Can you work these out from the model? Positions are in its coordinate system, mm. Face numbers are marked on the shaded views. A direction names the side the tool comes from. Round coordinates to 2 decimals unless told otherwise and drop trailing zeros. Loops run counter-clockwise (first coordinate to the right, second up) from the corner with the lowest first, then second, coordinate; pieces in that order, holes last. Notation, with made-up numbers: M 66.25,60.5 L 91.25,60.5 A5 cw 91.25,69.5 Z; hole C -18,57 d6. An arc over 180 degrees is marked long. Answer as CSV lines item,"result".
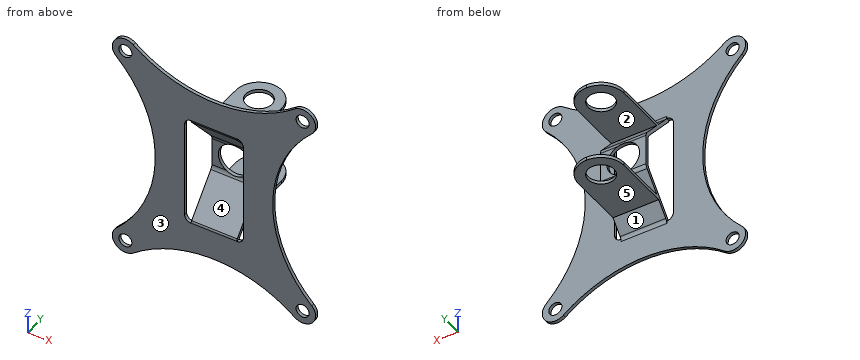
from build123d import *

# Parameters (mm, degrees)
BOSS_EXTRUDE1_DEPTH = 3.175
BOSS_EXTRUDE3_DEPTH = 22.225
SKETCH5_R           = 15.875
CUT_EXTRUDE1_DEPTH  = 35.925
SKETCH6_R           = 12.7
CUT_EXTRUDE2_DEPTH  = 79.375
FILLET1_R           = 6.35
SKETCH1_5_R         = 6.35
HOLES_DEPTH         = 92.0082


with BuildPart() as part:
    # Sketch1 → Boss-Extrude1 (new body)
    with BuildSketch(Plane(origin=(0, 0, 0), x_dir=(1, 0, 0), z_dir=(0, 1, 0))):
        with BuildLine():
            ThreePointArc((-78.393636364, 109.635915457), (-95.772926059, 108.027505481), (-95.134259734, 90.585636364))
            ThreePointArc((-95.134259734, 90.585636364), (-57.14685707, 0), (-95.134259734, -90.585636364))
            ThreePointArc((-95.134259734, -90.585636364), (-95.772926059, -108.027505481), (-78.393636364, -109.635915457))
            ThreePointArc((-78.393636364, -109.635915457), (0, -82.553070029), (78.393636364, -109.635915457))
            ThreePointArc((78.393636364, -109.635915457), (95.772926059, -108.027505481), (95.134259734, -90.585636364))
            ThreePointArc((95.134259734, -90.585636364), (57.14685707, 0), (95.134259734, 90.585636364))
            ThreePointArc((95.134259734, 90.585636364), (95.772926059, 108.027505481), (78.393636364, 109.635915457))
            ThreePointArc((78.393636364, 109.635915457), (0, 82.553070029), (-78.393636364, 109.635915457))
        make_face()
        with BuildLine():
            Line((-22.225, -53.975), (22.225, -53.975))
            ThreePointArc((22.225, -53.975), (26.715128061, -52.115128061), (28.575, -47.625))
            Line((28.575, -47.625), (28.575, 47.625))
            ThreePointArc((28.575, 47.625), (26.715128061, 52.115128061), (22.225, 53.975))
            Line((22.225, 53.975), (-22.225, 53.975))
            ThreePointArc((-22.225, 53.975), (-26.715128061, 52.115128061), (-28.575, 47.625))
            Line((-28.575, 47.625), (-28.575, -47.625))
            ThreePointArc((-28.575, -47.625), (-26.715128061, -52.115128061), (-22.225, -53.975))
        make_face(mode=Mode.SUBTRACT)
    extrude(amount=BOSS_EXTRUDE1_DEPTH)

    # Sketch4 → Boss-Extrude3 (add, symmetric)
    with BuildSketch(Plane(origin=(0, 0, 0), x_dir=(0, 0, -1), z_dir=(1, 0, 0))):
        with BuildLine():
            ThreePointArc((53.975, 0), (52.866902818, 0.199643612), (51.898159667, 0.773467316))
            Line((51.898159667, 0.773467316), (17.867550541, 30.203065368))
            ThreePointArc((17.867550541, 30.203065368), (15.930064238, 31.350712776), (13.713869875, 31.75))
            Line((13.713869875, 31.75), (-13.713869875, 31.75))
            ThreePointArc((-13.713869875, 31.75), (-15.930064238, 31.350712776), (-17.867550541, 30.203065368))
            Line((-17.867550541, 30.203065368), (-51.898159667, 0.773467316))
            ThreePointArc((-51.898159667, 0.773467316), (-52.866902818, 0.199643612), (-53.975, 0))
            Line((-53.975, 0), (-53.975, 3.175))
            Line((-53.975, 3.175), (-19.05, 33.378065368))
            ThreePointArc((-19.05, 33.378065368), (-17.112513698, 34.525712776), (-14.896319334, 34.925))
            Line((-14.896319334, 34.925), (14.896319334, 34.925))
            ThreePointArc((14.896319334, 34.925), (17.112513698, 34.525712776), (19.05, 33.378065368))
            Line((19.05, 33.378065368), (53.975, 3.175))
            Line((53.975, 3.175), (53.975, 0))
        make_face()
        Polygon((-39.6875, 91.0082), (-39.6875, 15.530799469), (-36.5125, 18.276532684), (-36.5125, 91.0082), align=None)
        Polygon((36.5125, 91.0082), (36.5125, 18.276532684), (39.6875, 15.530799469), (39.6875, 91.0082), align=None)
    extrude(amount=BOSS_EXTRUDE3_DEPTH, both=True)

    # Sketch5 → Cut-Extrude1 (cut, through all)
    with BuildSketch(Plane(origin=(0, 34.925, 0), x_dir=(1, 0, 0), z_dir=(0, 1, 0))):
        Circle(SKETCH5_R)
    extrude(amount=-CUT_EXTRUDE1_DEPTH, mode=Mode.SUBTRACT)

    # Sketch6 → Cut-Extrude2 (cut)
    with BuildSketch(Plane(origin=(0, 0, -39.6875), x_dir=(-1, 0, 0), z_dir=(0, 0, -1))):
        with Locations((0, 68.7832)):
            Circle(SKETCH6_R)
        with BuildLine():
            ThreePointArc((-22.225, 68.7832), (-15.715448152, 84.498648271), (1.69e-07, 91.0082))
            Line((1.69e-07, 91.0082), (-22.225, 91.0082))
            Line((-22.225, 91.0082), (-22.225, 68.7832))
        make_face()
        with BuildLine():
            Line((22.225, 68.7832), (22.225, 91.0082))
            Line((22.225, 91.0082), (1.69e-07, 91.0082))
            ThreePointArc((1.69e-07, 91.0082), (15.715448271, 84.498648152), (22.225, 68.7832))
        make_face()
    extrude(amount=-CUT_EXTRUDE2_DEPTH, mode=Mode.SUBTRACT)

    # Fillet1
    fillet1_edges = [part.edges().sort_by_distance(p)[0] for p in [
        (0, 3.175, -53.975),
        (0, 3.175, 53.975),
    ]]
    fillet(fillet1_edges, radius=FILLET1_R)

    # Sketch1<5> → holes (cut, through all)
    with BuildSketch(Plane(origin=(0, 0, 0), x_dir=(1, 0, 0), z_dir=(0, 1, 0))):
        with Locations((-86.233, 99.6442)):
            Circle(SKETCH1_5_R)
        with Locations((86.233, 99.6442)):
            Circle(SKETCH1_5_R)
        with Locations((86.233, -99.6442)):
            Circle(SKETCH1_5_R)
        with Locations((-86.233, -99.6442)):
            Circle(SKETCH1_5_R)
    extrude(amount=HOLES_DEPTH, mode=Mode.SUBTRACT)


solid = part.part
Item 1: On a 3-axis mill with a long thin cutter (end or side, diameter ignored), from which of +Z, -Z, +X, -X, +Y, -Y can I reach the whole of each face in a straight line? I mean the marked faces 1 and 2. Say none if no direction works.
Output:
face 1,"-Z, +X, -X, +Y"
face 2,"+X, -X, +Y"
Item 2: If we section it at C-C on x = -62: Write out the boundary of the cut face in (y, z) (3 decimals), then the cut area to 3 significant figures.
Output:
outline,"M 0,-98.715 L 3.175,-98.715 L 3.175,-34.773 L 0,-34.773 Z; M 0,34.773 L 3.175,34.773 L 3.175,98.715 L 0,98.715 Z"
area,"406 mm2"
Item 3: We'd pull the mould along Z, two halves only. Please class the marked faces 3, 4 and 5: released by +Z, released by -Z, zero draft, split by the parting line, or undercut.
Output:
face 3,"zero draft"
face 4,"undercut"
face 5,"released by -Z"
Item 4: If we section it at A-A on z = 0: Write out the boundary of the cut face in (x, y) (3 decimals), then the cut area to 3 significant figures.
Output:
outline,"M -57.147,0 L -28.575,0 L -28.575,3.175 L -57.147,3.175 Z; M -22.225,31.75 L -15.875,31.75 L -15.875,34.925 L -22.225,34.925 Z; M 15.875,31.75 L 22.225,31.75 L 22.225,34.925 L 15.875,34.925 Z; M 28.575,0 L 57.147,0 L 57.147,3.175 L 28.575,3.175 Z"
area,"222 mm2"
Item 5: If we section it at D-D on x = 61.5: Write out the boundary of the cut face in (y, z) (3 decimals).
Output:
outline,"M 0,-98.437 L 3.175,-98.437 L 3.175,-32.966 L 0,-32.966 Z; M 0,32.966 L 3.175,32.966 L 3.175,98.437 L 0,98.437 Z"
Item 6: Will these pins go through, and if not, where does the flat tip stop? pin 1 (14.5 mm diameter, centred on x = 86.23, z = -99.64, fed in from -Y); pin 2 (2.5 mm diameter, centred on y = 2, z = -20.5, fed in from -X); pin 3 (13.5 mm diameter, centred on x = -10.5, y = 42.5, fed in from +Z); pin 4 (3 mm diameter, centred on y = 35, z = -40.5, fed in from -X) (3 decimals).
Output:
pin 1,"stops at y = 0"
pin 2,"stops at x = -59.02"
pin 3,"stops at z = 39.69"
pin 4,"stops at x = -22.225"
Item 7: If we section it at B-B on x = 83.5: Write out the boundary of the cut face in (y, z) (3 decimals).
Output:
outline,"M 0,-112.047 L 3.175,-112.047 L 3.175,-105.376 L 0,-105.376 Z; M 0,-93.912 L 3.175,-93.912 L 3.175,-77.455 L 0,-77.455 Z; M 0,77.455 L 3.175,77.455 L 3.175,93.912 L 0,93.912 Z; M 0,105.376 L 3.175,105.376 L 3.175,112.047 L 0,112.047 Z"
Item 8: If I drill on line 1 along Z through (x, y) = (0, 33.7) (1 decimal); line 2 along Z through (x, y) = (19, 72.5); line 3 along Z through (x, y) = (0, 33.9) (1 decimal), over which ranges is the centre line in solid material (lowest first)? Write a range as from..to.
Output:
line 1,"z = -39.7..-36.5, -18.6..-15.9, 15.9..18.6, 36.5..39.7"
line 2,"z = -39.69..-36.51, 36.51..39.69"
line 3,"z = -39.7..-36.5, -18.4..-15.9, 15.9..18.4, 36.5..39.7"
